Answer from the drawing. Dimensions are ordinates in mm from the lowest x, y and z of the part. Give positions to 0.01 mm unless a question says otherwise; leave off trailing zeros. Loops run counter-clockwise (first coordinate to the right, second up) from the corner with the lowest first, then second, coordinate; pieces in that order, holes last. Notation, with made-up numbers: (55, -17) - (70, -17) arc R30 ccw to (70, 18) - close; hole circle Ø9 at (74, 58). An arc over 180 degrees is marked (long way). Answer as CSV lines item,"result". Start each with the question number.
1) Flat-ended cylindrical pins translate along their axes: pin 1 (1 mm diameter, centred on x = 21.5, z = 0.5, fed in from +Y); pin 2 (1.6 mm diameter, centred on y = 49, z = 1, fed in from -X); pin 3 (1.6 mm diameter, centred on x = 27, z = 1, fed in from -Y). Find the tip coordinate at first contact, or state that the pin passes through.
2) Find the intervals of material crossed by line 1 along Y through (x, z) = (47, 1.6); line 2 along X through (y, z) = (15, 3.15); line 3 along X through (y, z) = (15, 1.45), in increasing order.
3) A cutting plane is placed at A-A (y = 59). Determine the outline of the cut face in (x, z), and give its area (3 significant figures).
4) A cutting plane is placed at B-B (x = 48.5). Determine the outline of the cut face in (y, z), and give its area (3 significant figures).
5) A cutting plane is placed at C-C (y = 123). Determine the outline of the cut face in (x, z).
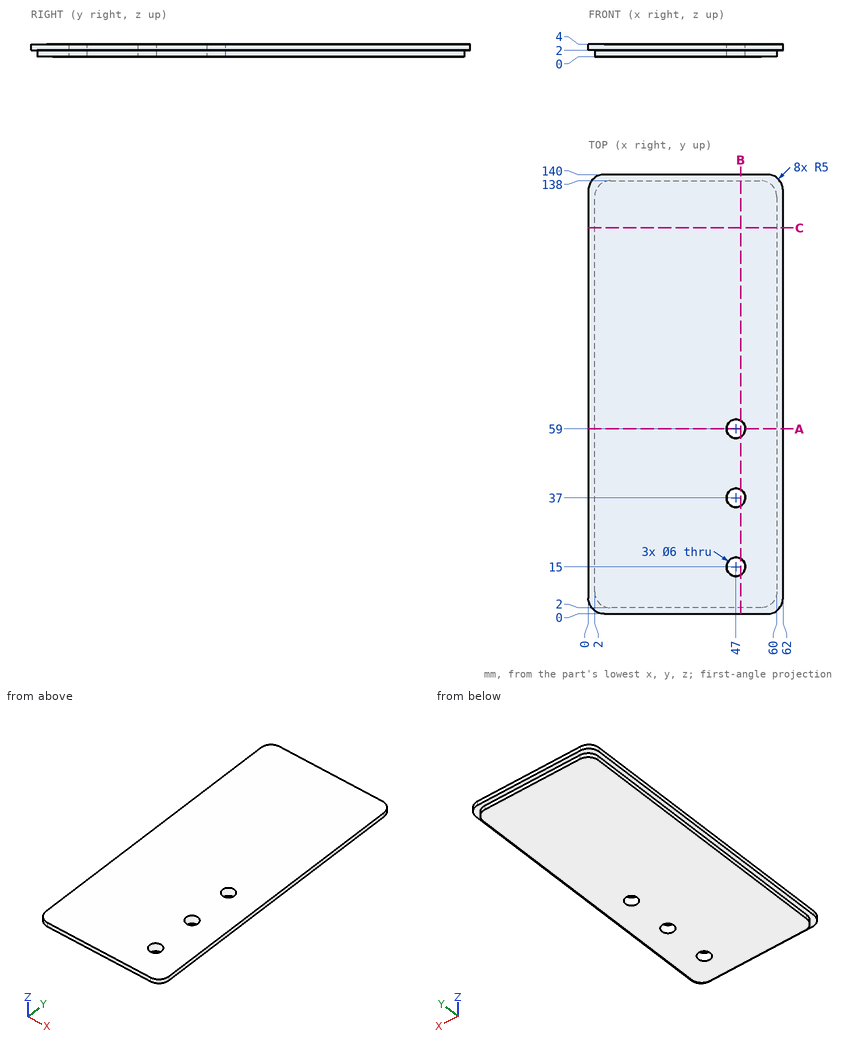
Ans:
1,pin 1,"y = 138"
1,pin 2,"x = 2"
1,pin 3,"y = 2"
2,line 1,"2 to 12, 18 to 34, 40 to 56, 62 to 138"
2,line 2,"0 to 44, 50 to 62"
2,line 3,"2 to 44, 50 to 60"
3,outline,"(0, 2) - (2, 2) - (2, 0) - (44, 0) - (44, 4) - (0, 4) - close; (50, 0) - (60, 0) - (60, 2) - (62, 2) - (62, 4) - (50, 4) - close"
3,area,"216 mm2"
4,outline,"(0, 2) - (2, 2) - (2, 0) - (12.4, 0) - (12.4, 4) - (0, 4) - close; (17.6, 0) - (34.4, 0) - (34.4, 4) - (17.6, 4) - close; (39.6, 0) - (56.4, 0) - (56.4, 4) - (39.6, 4) - close; (61.6, 0) - (138, 0) - (138, 2) - (140, 2) - (140, 4) - (61.6, 4) - close"
4,area,"490 mm2"
5,outline,"(0, 2) - (2, 2) - (2, 0) - (60, 0) - (60, 2) - (62, 2) - (62, 4) - (0, 4) - close"
